Answer from the drawing. Dimensions are ordinates in mm from the lowest x, y and z of the part. Round coordinates to 2 decimals unless told otherwise and drop trailing zeros. Order: outer loops, then holes, each group sorted by start corner. A loop starts at its lowest first (then second) coordinate and runs counter-clockwise, first axis right, second up. Notation, with made-up numbers: M 17.5,48.25 L 74.5,48.25 A30 cw 74.5,70.25 Z; hole C -35.75,0.5 d10. An arc over 180 degrees is marked long. Write item = value, one per line. Start each with the question number.
(1) A cutting plane is placed at C-C, the plane y = 106.5. Determine the outline of the cut face in (x, z), and give its area (3 significant figures).
(2) Each of these flat-tipped pins is pushed along its axis until it touches: pin 1 (4 mm diameter, centred on x = 24.5, y = 177.5, fed in from -Z); pin 2 (3 mm diameter, centred on y = 261.5, z = 74.5, fed in from -X). Where does it stop, or does it pass through?
(3) Straight lines are drawn through the part: probe 1 along Z at (x, y) = (35.5, 258); probe 2 along Y at (x, z) = (6, 21.5). For each, find the intervals that lie inside material, in ascending order. Write a range as from..to.
(4) A cutting plane is placed at A-A, the plane x = 31.75. Determine the outline of the cut face in (y, z), and give its area (3 significant figures).
(5) A cutting plane is placed at B-B, the plane y = 30. Determine the outline of the cut face in (x, z), and give its area (3 significant figures).
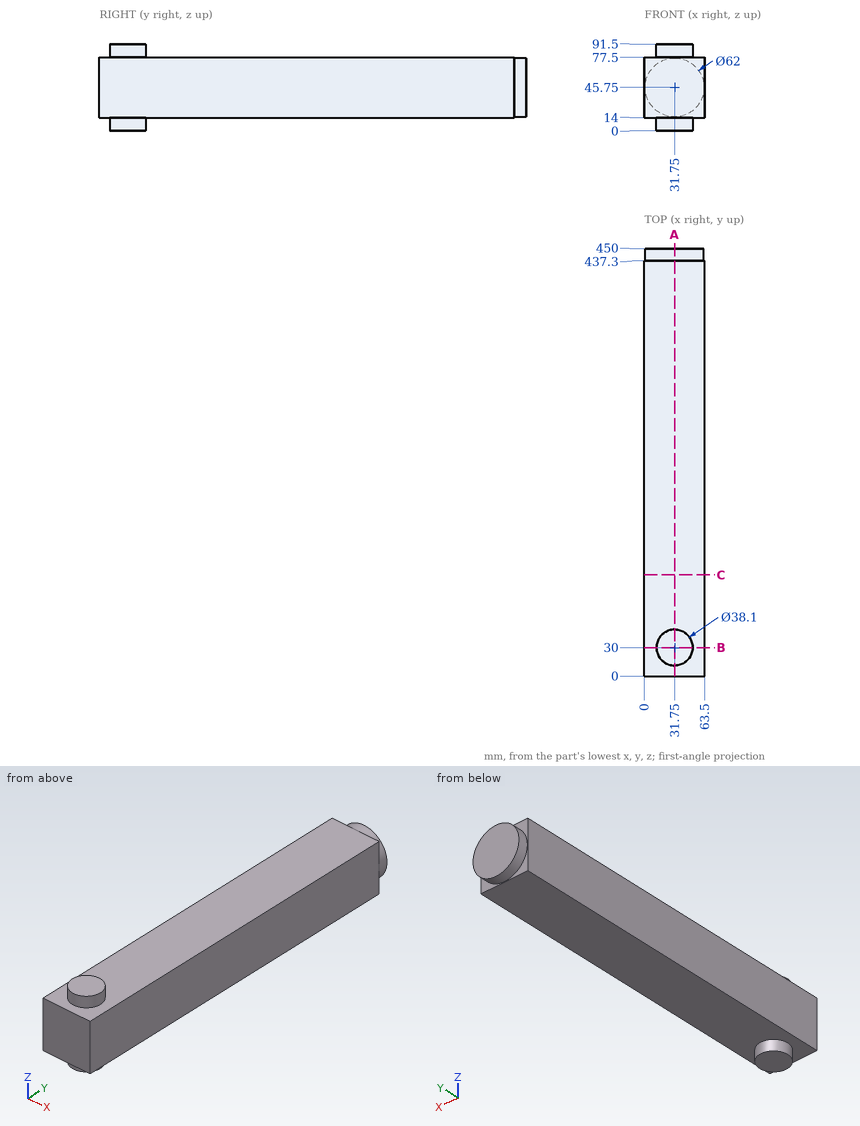
Reported:
q1.outline = M 0,14 L 63.5,14 L 63.5,77.5 L 0,77.5 Z
q1.area = 4,030 mm²
q2.pin_1 = 14
q2.pin_2 = 0
q3.probe_1 = 14..77.5
q3.probe_2 = 0..437.3
q4.outline = M 0,14 L 10.95,14 L 10.95,0 L 49.05,0 L 49.05,14 L 437.3,14 L 437.3,14.75 L 450,14.75 L 450,76.75 L 437.3,76.75 L 437.3,77.5 L 49.05,77.5 L 49.05,91.5 L 10.95,91.5 L 10.95,77.5 L 0,77.5 Z
q4.area = 29,600 mm²
q5.outline = M 0,14 L 12.7,14 L 12.7,0 L 50.8,0 L 50.8,14 L 63.5,14 L 63.5,77.5 L 50.8,77.5 L 50.8,91.5 L 12.7,91.5 L 12.7,77.5 L 0,77.5 Z
q5.area = 5,100 mm²
